Autodesk Inventor part; units mm, degrees
ref_plane "YZ Plane" through (0, 0, 0) normal (1, 0, 0) x (0, 1, 0)
ref_plane "XZ Plane" through (0, 0, 0) normal (0, 1, 0) x (-1, 0, 0)
ref_plane "XY Plane" through (0, 0, 0) normal (0, 0, 1) x (1, 0, 0)
sketch "Sketch1" plane through (0, 0, 0) normal (0, 0, 1) x (1, 0, 0)
  line L0 (25.4, 0) -> (-25.4, 0) construction
  line L1 (25.4, 0) -> (25.4, -38.1)
  line L2 (-25.4, -38.1) -> (-25.4, 0)
  line L3 (0, 57.7256) -> (0, -54.0709) construction
  line L4 (-25.4, -38.1) -> (25.4, -38.1)
  line L5 (25.4, 0) -> (8.4711, 32.9299)
  arc A0 (6.9296, 22.04) -> (3.175, 19.5947) centre (0, 28.575) ccw
  line L6 (-8.4711, 32.9299) -> (-25.4, 0)
  line L7 (15.8117, 4.7625) -> (6.9296, 22.04)
  line L8 (3.175, 19.5947) -> (3.175, 4.7625)
  line L9 (3.175, 4.7625) -> (15.8117, 4.7625)
  arc A1 (3.175, 19.5947) -> (6.9296, 22.04) centre (0, 28.575) ccw
  line L10 (-15.8117, 4.7625) -> (-6.9296, 22.04)
  line L11 (-3.175, 19.5947) -> (-3.175, 4.7625)
  line L12 (-3.175, 4.7625) -> (-15.8117, 4.7625)
  arc A2 (-6.9296, 22.04) -> (-3.175, 19.5947) centre (0, 28.575) ccw
  point P0 (0, 0)
  point P1 (0, 0)
  point P2 (-3.175, 19.5947)
  point P3 (-6.9296, 22.04)
  dimension "d112" = 28.575
  dimension "d113" = 9.525
  dimension "d114" = 50.8
  dimension "d115" = 38.1
  dimension "d117" = 6.35
  dimension "d118" = 4.7625
  dimension "d119" = 6.35
extrude "Extrusion2" add sketch "Sketch1" along normal mid plane 6.35 contours L1 L4 L2 L6 A0 L10 L12 L11 L8 L9 L7 L5 | A0 A1
sketch "Sketch3" plane through (0, 0, -3.175) normal (0, 0, -1) x (-1, 0, 0)
  line L0 (-35.56, 0) -> (35.56, 0) construction
  line L1 (0, -53.34) -> (0, 53.34) construction
  line L2 (12.7, -3.175) -> (-12.7, -3.175) construction
  line L3 (12.7, -15.875) -> (-12.7, -15.875) construction
  line L4 (12.7, -28.575) -> (-12.7, -28.575) construction
  point P0 (0, 0)
  point P1 (0, -3.175)
  point P2 (0, -15.875)
  point P3 (0, -28.575)
  dimension "d43" = 25.4
  dimension "d45" = 3.175
  dimension "d107" = 12.7
hole "Hole2" at (12.7, -3.175, -3.175) at (-12.7, -3.175, -3.175) at (0, -3.175, -3.175) at (12.7, -15.875, -3.175) at (0, -15.875, -3.175) at (-12.7, -15.875, -3.175) at (12.7, -28.575, -3.175) at (0, -28.575, -3.175) at (-12.7, -28.575, -3.175) direction (0, 0, 1) diameter 5.1054 end through all
sketch "Sketch7" plane through (0, 0, -3.175) normal (0, 0, 1) x (1, 0, 0)
  arc A0 (8.4711, 32.9299) -> (-8.4711, 32.9299) centre (0, 28.575) ccw construction
  point P0 (0, 0)
hole "Hole4" at (0, 28.575, -3.175) direction (0, 0, 1) diameter 7.9375 end through all
fillet "Fillet5" radius 3.175 2 edges at (-25.4, -38.1, 0) (25.4, -38.1, 0)
fillet "Fillet7" radius 1.5875 8 edges at (-15.8117, 4.7625, 0) (-6.9296, 22.04, 0) (-3.175, 19.5947, 0) (-3.175, 4.7625, 0) (3.175, 4.7625, 0) (3.175, 19.5947, 0) (6.9296, 22.04, 0) (15.8117, 4.7625, 0)
fillet "Fillet9" radius 25.4 2 edges at (25.4, 0, 0) (-25.4, 0, 0)
equation "\"BendRadius\" = Thickness"
equation "\"BendReliefWidth\" = Thickness"
equation "\"BendReliefDepth\" = 0.5 * Thickness"
equation "\"CornerReliefSize\" = 4 * Thickness"
equation "\"MinimumRemnant\" = 2 * Thickness"
equation "\"TransitionRadius\" = BendRadius"
equation "\"JacobiRadiusSize\" = BendRadius"
equation "\"GapSize\" = Thickness"
properties part number "PLATE,SIDE,PULLEY,MOUNT,TOP,ELEVATORR" material "Aluminum 7075"
Work out the finished part from the listing and answer in its coordinate system (mm). A direction names the side the tool comes from. Round coordinates to 2 decimals unless told otherwise and drop trailing zeros. Write each loop counter-clockwise with the first axis right and the second up, starting at its lowest first coordinate (ties: lowest second). Pieces come first, ordered by that corner, then holes.
1) Consider probe 1 along Y at (x, z) = (0, 0.5); probe 2 along X at (y, z) = (13, -1) (3 decimals); probe 3 along X at (y, z) = (11, 1.75) (3 decimals). Determine where each line is inside the solid, lowest interval first.
2) Flat-ended cylindrical pins translate along their axes: P1, Ø3, axis at x = 10.5, z = -0.5, coming from the +Y side; P2, Ø3, axis at x = -12.7, y = -15.875, coming from the +Z side; P3, Ø6.5, axis at x = 12.7, y = -15.875, coming from the -Z side (3 decimals); P4, Ø3, axis at y = 15.5, z = 0, coming from the +X side. Find the tip coordinate at first contact, or state that the pin passes through.
3) Determine the mould class of faces 3 (the face through (-11.285, 13.568, -0.044)), 4 (the face through (4.83, 20.365, -0.044)), 5 (the face through (-0.1, 38.1, 0)), 6 (the face through (-24.45, -37.19, -0.04)) for opening direction Y: pulls with the +Y half, pulls with the -Y half, needs draft (parallel to the pull), parting line crosses it, or undercut.
4) A cutting plane is placed at B-B on y = -30. Determine the outline of the cut face in (x, z) (3 decimals).
5) A cutting plane is placed at C-C on y = 15. Determine the outline of the cut face in (x, z) (3 decimals), and give its area (3 significant figures).
6) A cutting plane is placed at A-A on x = 0. Determine the outline of the cut face in (y, z) (3 decimals).
7) Which of the six approach directions +Z, -Z, +X, -X, +Y, -Y give full straight-line access (tool end or side, diameter ignored) to faces 1 (the face through (-14.55, 5.5, -0.04)), 2 (the face through (0, -8, 3.175))?
8) A cutting plane is placed at D-D on y = 27. Determine the outline of the cut face in (x, z) (3 decimals).
Entries:
1. probe 1: y = -38.1 to -31.13, -26.02 to -18.43, -13.32 to -5.73, -0.62 to 24.61, 32.54 to 38.1
1. probe 2: x = -18.717 to -11.577, -3.175 to 3.175, 11.577 to 18.717
1. probe 3: x = -19.745 to -12.605, -3.175 to 3.175, 12.605 to 19.745
2. P1: stops at y = 31.9
2. P2: passes through
2. P3: stops at z = -3.175
2. P4: stops at x = 18.2
3. face 3: undercut
3. face 4: undercut
3. face 5: pulls with the +Y half
3. face 6: pulls with the -Y half
4. outline: (-25.4, -3.175) - (-14.818, -3.175) - (-14.818, 3.175) - (-25.4, 3.175) - close; (-10.582, -3.175) - (-2.118, -3.175) - (-2.118, 3.175) - (-10.582, 3.175) - close; (2.118, -3.175) - (10.582, -3.175) - (10.582, 3.175) - (2.118, 3.175) - close; (14.818, -3.175) - (25.4, -3.175) - (25.4, 3.175) - (14.818, 3.175) - close
5. outline: (-17.689, -3.175) - (-10.549, -3.175) - (-10.549, 3.175) - (-17.689, 3.175) - close; (-3.175, -3.175) - (3.175, -3.175) - (3.175, 3.175) - (-3.175, 3.175) - close; (10.549, -3.175) - (17.689, -3.175) - (17.689, 3.175) - (10.549, 3.175) - close
5. area: 131 mm2
6. outline: (-38.1, -3.175) - (-31.128, -3.175) - (-31.128, 3.175) - (-38.1, 3.175) - close; (-26.022, -3.175) - (-18.428, -3.175) - (-18.428, 3.175) - (-26.022, 3.175) - close; (-13.322, -3.175) - (-5.728, -3.175) - (-5.728, 3.175) - (-13.322, 3.175) - close; (-0.622, -3.175) - (24.606, -3.175) - (24.606, 3.175) - (-0.622, 3.175) - close; (32.544, -3.175) - (38.1, -3.175) - (38.1, 3.175) - (32.544, 3.175) - close
7. face 1: +Z, -Z
7. face 2: +Z, +X, -X, +Y, -Y
8. outline: (-11.52, -3.175) - (-3.643, -3.175) - (-3.643, 3.175) - (-11.52, 3.175) - close; (3.643, -3.175) - (11.52, -3.175) - (11.52, 3.175) - (3.643, 3.175) - close
